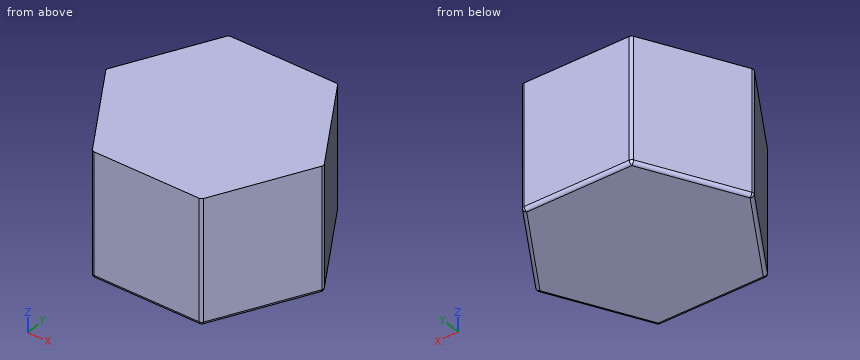
```python
from build123d import *

# Parameters (mm, degrees)
F1_DEPTH = 37.5
F2_R     = 1


with BuildPart() as f1:
    # F0 (on Top) → F1 (new body)
    with BuildSketch(Plane.XY):
        Polygon((-15.732795, -27.25), (15.732795, -27.25), (31.46559, 0), (15.732795, 27.25), (-15.732795, 27.25), (-31.46559, 0), align=None)
    extrude(amount=F1_DEPTH)

    # F2
    f2_edges = [f1.edges().sort_by_distance(p)[0] for p in [
        (0, -27.25, 0),
        (23.599192, -13.625, 0),
        (23.599192, 13.625, 0),
        (0, 27.25, 0),
        (-23.599192, 13.625, 0),
        (-23.599192, -13.625, 0),
        (15.732795, -27.25, 18.75),
        (31.46559, 0, 18.75),
        (-15.732795, -27.25, 18.75),
        (-31.46559, 0, 18.75),
        (-15.732795, 27.25, 18.75),
        (15.732795, 27.25, 18.75),
    ]]
    fillet(f2_edges, radius=F2_R)


solid = f1.part
```
Could you check a few things on this model? Use its own coordinates, in mm. Round coordinates to 2 decimals unless told otherwise and drop trailing zeros. Write each loop counter-clockwise with the first axis right and the second up, starting at its lowest first coordinate (ties: lowest second). Pieces come first, ordered by that corner, then holes. Notation, with made-up numbers: M -38.75,32.25 L 20.25,32.25 A23 cw 20.25,50.25 Z; hole C -12,53.25 d5. An arc over 180 degrees is marked long. Write each question's results on one line, items separated by ' | '. Start each with the question number.
1. I'm going to push flat-ended pins straight in: pin 1 Ø6 at (y, z) = (13, 33.5) entering from -X; pin 2 Ø4 at (y, z) = (7, 5.5) entering from -X; pin 3 Ø8 at (x, z) = (-19.5, 19.5) entering from -Y. Where does each tip first touch, or does it pass through?
2. Imagine slicing it at A-A on z = 29. List the corners of the cut face in (x, y) for me.
3. I need wall thicknesses on L1, parallel to Z at x = 25, y = 9.5; L2, parallel to X at y = -7.5, z = 11.5; L3, parallel to X at y = -17.5, z = 34.5. Which ranges of each line are inside material? Lowest first, please. Write a range as from..to.
Result sheet:
1) pin 1: stops at x = -25.69 | pin 2: stops at x = -28.58 | pin 3: stops at y = -27.19
2) outline: M -31.18,-0.5 L -16.02,-26.75 A1 ccw -15.16,-27.25 L 15.16,-27.25 A1 ccw 16.02,-26.75 L 31.18,-0.5 A1 ccw 31.18,0.5 L 16.02,26.75 A1 ccw 15.16,27.25 L -15.16,27.25 A1 ccw -16.02,26.75 L -31.18,0.5 A1 ccw Z
3) L1: z = 0.01..37.5 | L2: x = -27.14..27.14 | L3: x = -21.36..21.36
